Work out the finished part from the listing and answer in its coordinate system (mm). A direction names the side the tool comes from. Give positions to 0.01 mm unless a question says otherwise; leave off trailing zeros. Loops run counter-clockwise (first coordinate to the right, second up) from the corner with the lowest first, then second, coordinate; pieces in that order, holes last. Notation, with made-up numbers: M -5.75,70.5 L 19.25,70.5 A20 ccw 19.25,105.5 Z; hole C 61,89 d2. An arc over 180 degrees is marked long. Write item = value, one per line. Start each with the question number.
1. Section A-A on z = 5.5 is taken. Determine the outline of the cut face in (x, y), plus the area to 3 significant figures.
2. Consider L1, parallel to Y at x = 3, z = 8.3; L2, parallel to X at y = 9, z = 7.85; L3, parallel to X at y = 8.5, z = 8.75. Determine where each line is inside the solid, lowest interval first. Write a range as [from, to].
3. For faces 4 (the face through (8, 6, 0)), 5 (the face through (3, 9.8, 7.5)), determine the directions among +Z, -Z, +X, -X, +Y, -Y from which every point of the face is accessible in a straight line to the end or side of a thin tool.
4. A flat-ended cylindrical pin translates along its axis: pin 1 Ø2.5 at (x, y) = (3, 3) entering from -Z. Find the tip coordinate at first contact, or state that the pin passes through.
5. The mould has two halves that part along X. Classify faces 1 (the face through (17, 6, 5)), 2 (the face through (9, 6, 10)), 3 (the face through (3.71, 2.63, 7.46)): released by +X, released by -X, zero draft, split by the parting line, or undercut.
Autodesk Fusion 360 part; units mm, degrees
sketch "Sketch1" plane through (0, 0, 0) normal (0, 1, 0) x (1, 0, 0)
  line L0 (0, 0) -> (17, 0)
  line L1 (17, 0) -> (17, -10)
  line L2 (17, -10) -> (0, -10)
  line L3 (0, -10) -> (0, 0)
  dimension "d1" = 17
  dimension "d2" = 10
extrude "Extrude1" add sketch "Sketch1" along normal blind 12
sketch "Sketch2" plane through (0, 0, 10) normal (0, 0, 1) x (1, 0, 0)
  line L0 (0, 0) -> (17, 0)
  line L1 (17, 0) -> (17, 12)
  line L2 (17, 12) -> (0, 12)
  line L3 (0, 12) -> (0, 0)
  point P0 (3, 3)
  point P1 (3, 9)
  dimension "d5" = 3
  dimension "d6" = 3
  dimension "d7" = 6
hole "Hole1" at (3, 3, 10) direction (0, 0, -1) diameter 1.6 depth 5 tip angle 118
hole "Hole2" at (3, 9, 10) direction (0, 0, -1) diameter 1.6 depth 5 tip angle 118
Verdict:
q1.outline = M 0,0 L 17,0 L 17,12 L 0,12 Z; hole C 3,3 d1.6; hole C 3,9 d1.6
q1.area = 200 mm2
q2.L1 = [0, 2.2], [3.8, 8.2], [9.8, 12]
q2.L2 = [0, 2.2], [3.8, 17]
q2.L3 = [0, 2.38], [3.62, 17]
q3.face_4 = -Z, +X, -X, +Y, -Y
q3.face_5 = +Z
q4.pin_1 = 0
q5.face_1 = released by +X
q5.face_2 = zero draft
q5.face_3 = undercut
